Can you work these out from the drawing? Everything is in mm from the part's minimum corner. Coordinates: 2 decimals unless noted, no trailing zeros. Order: outer loops, then holes, each group sorted by start corner. A loop starts at its lowest first (then second) coordinate and runs counter-clockwise, first axis right, second up. Notation, with made-up numbers: (35, 5.5) -> (39, 5.5) arc R18 ccw to (39, 30.5) -> close; hole circle Ø2 at (37.25, 50.5). An arc over 180 degrees is marked (long way). Write item = value, one per line. Start each with the question number.
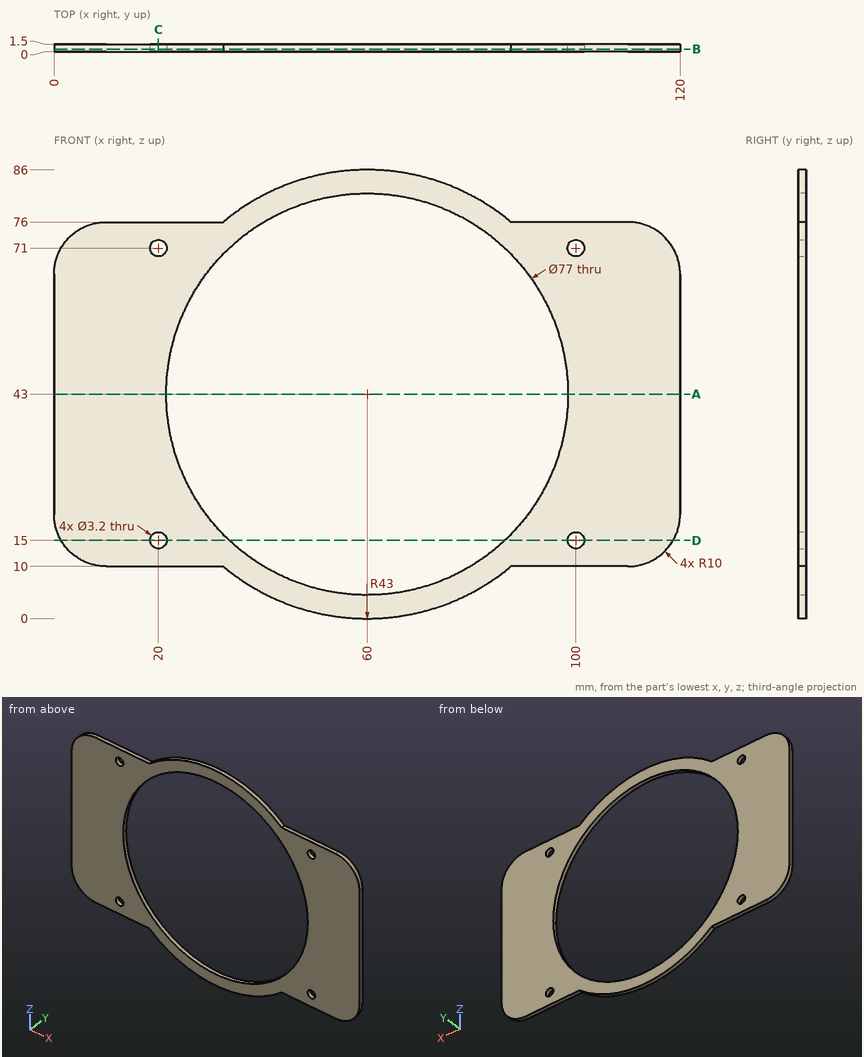
(1) Imagine slicing it at B-B (y = 0.5). Write out the boundary of the cut face in (x, z).
(2) Imagine slicing it at C-C (x = 20). Write out the boundary of the cut face in (y, z).
(3) For P1, Ø0.8, axis at x = 95.5, y = 0.5, coming from the -Z side; P2, Ø3, axis at x = 100, z = 71, coming from the +Y side, each with a flat end and sliding along its axis, tell me the tip position at first contact or that it passes through.
(4) Imagine slicing it at D-D (z = 15). Write out the boundary of the cut face in (x, y).
(5) Imagine slicing it at A-A (z = 43). Write out the boundary of the cut face in (x, y), plus the area to 3 significant figures.
(6) If I drill on L1, parallel to Z at x = 20, y = 0.55; L2, parallel to Z at x = 61, y = 0.35; L3, parallel to X at y = 0.9, z = 43, over which ranges is the centre line in solid material (lowest first)? Write a range as from..to.
Result set:
q1.outline = (0, 20) arc R10 ccw to (10, 10) -> (32.43, 10) arc R43 ccw to (87.57, 10) -> (110, 10) arc R10 ccw to (120, 20) -> (120, 66) arc R10 ccw to (110, 76) -> (87.57, 76) arc R43 ccw to (32.43, 76) -> (10, 76) arc R10 ccw to (0, 66) -> close; hole circle Ø3.2 at (20, 15); hole circle Ø3.2 at (20, 71); hole circle Ø77 at (60, 43); hole circle Ø3.2 at (100, 15); hole circle Ø3.2 at (100, 71)
q2.outline = (0, 10) -> (1.5, 10) -> (1.5, 13.4) -> (0, 13.4) -> close; (0, 16.6) -> (1.5, 16.6) -> (1.5, 69.4) -> (0, 69.4) -> close; (0, 72.6) -> (1.5, 72.6) -> (1.5, 76) -> (0, 76) -> close
q3.P1 = 10
q3.P2 = through
q4.outline = (1.34, 0) -> (18.4, 0) -> (18.4, 1.5) -> (1.34, 1.5) -> close; (21.6, 0) -> (33.58, 0) -> (33.58, 1.5) -> (21.6, 1.5) -> close; (86.42, 0) -> (98.4, 0) -> (98.4, 1.5) -> (86.42, 1.5) -> close; (101.6, 0) -> (118.66, 0) -> (118.66, 1.5) -> (101.6, 1.5) -> close
q5.outline = (0, 0) -> (21.5, 0) -> (21.5, 1.5) -> (0, 1.5) -> close; (98.5, 0) -> (120, 0) -> (120, 1.5) -> (98.5, 1.5) -> close
q5.area = 64.5 mm2
q6.L1 = 10..13.4, 16.6..69.4, 72.6..76
q6.L2 = 0.01..4.51, 81.49..85.99
q6.L3 = 0..21.5, 98.5..120
